Design review of the part shown in the three views and the two pictorial views. Dimensions are in mm from the part's minimum x, y and z. A direction names the side the tool comes from. Give positions to 0.01 mm unless a question says otherwise; leave off trailing zeros. Loops run counter-clockwise (first coordinate to the right, second up) from the corner with the lowest first, then second, coordinate; pieces in that order, holes last.
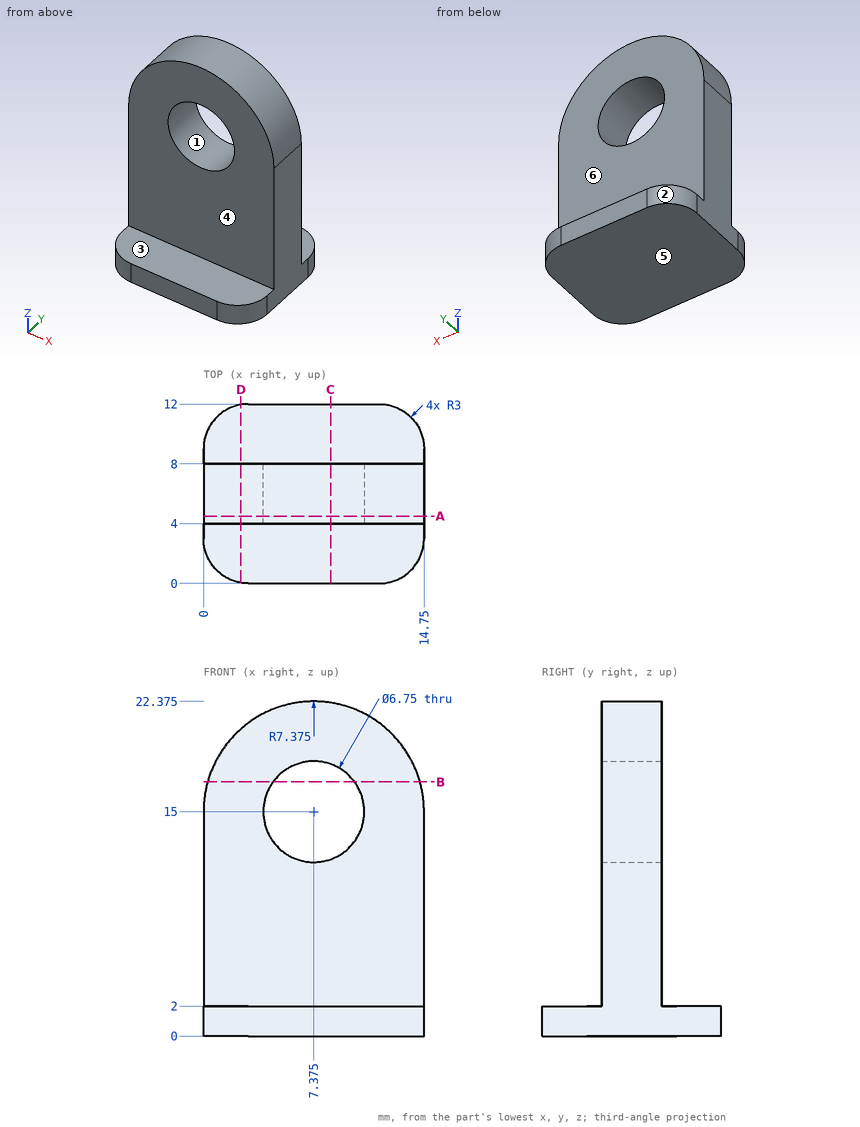
Q1. Mouldability with a two-part tool opening along Z and no side actions: class the marked faces 1, 2 and 3 as +Z half, -Z half, draft (parallel to the pull), parting line (faces both ways), or undercut.
Answers:
face 1: undercut
face 2: draft
face 3: +Z half
Q2. Consider section B-B on z = 17. Give the boundary of the cut face in (x, y).
Answers:
outline: (0.28, 4) - (4.66, 4) - (4.66, 8) - (0.28, 8) - close; (10.09, 4) - (14.47, 4) - (14.47, 8) - (10.09, 8) - close
Q3. For probe 1 along Z at (x, y) = (14.25, 3.75); probe 2 along Y at (x, z) = (9.25, 19.5); probe 3 along X at (y, z) = (7.75, 15.25), list the stretches that pass through material, from the lowest coordinate up.
Answers:
probe 1: z = 0 to 2
probe 2: y = 4 to 8
probe 3: x = 0 to 4.01, 10.74 to 14.75
Q4. Consider section A-A on y = 4.5. Give the boundary of the cut face in (x, z) (3 decimals), plus the area to 3 significant figures.
Answers:
outline: (0, 0) - (14.75, 0) - (14.75, 15) arc R7.375 ccw to (0, 15) - close; hole circle Ø6.75 at (7.375, 15)
area: 271 mm2
Q5. Consider section D-D on x = 2.5. Give the boundary of the cut face in (y, z).
Answers:
outline: (0.04, 0) - (11.96, 0) - (11.96, 2) - (8, 2) - (8, 20.53) - (4, 20.53) - (4, 2) - (0.04, 2) - close
Q6. Machinability: for the marked faces 4, 5 and 6, which of the approach directions +Z, -Z, +X, -X, +Y, -Y give a long, thin tool a straight path to every point of the face, cutting with its end or side? Answer none if there is none.
Answers:
face 4: +Z, +X, -X, -Y
face 5: -Z, +X, -X, +Y, -Y
face 6: +Z, +X, -X, +Y
Q7. Consider section C-C on x = 8.5. Give the boundary of the cut face in (y, z), plus the area to 3 significant figures.
Answers:
outline: (0, 0) - (12, 0) - (12, 2) - (8, 2) - (8, 11.82) - (4, 11.82) - (4, 2) - (0, 2) - close; (4, 18.18) - (8, 18.18) - (8, 22.29) - (4, 22.29) - close
area: 79.7 mm2
Q8. For pin 1 Ø4 at (x, z) = (4, 11.5) entering from -Y; pin 2 Ø3 at (y, z) = (3.5, 17) entering from -X; pin 3 Ø8 at (x, z) = (2.5, 19.5) entering from +Y, all flat-tipped, find the tip position at first contact; note any pin that passes through.
Answers:
pin 1: stops at y = 4
pin 2: stops at x = 0.02
pin 3: stops at y = 8
